Print and shaded views of the part. All mm, measured from the part's lowest x, y and z. Round coordinates to 2 decimals unless told otherwise and drop trailing zeros. Write each loop counter-clockwise with the first axis right and the second up, starting at its lowest first coordinate (ties: lowest second). Pieces come first, ordered by that corner, then holes. Notation, with made-up numbers: (29.25, -7.5) - (86.25, -7.5) arc R10 cw to (86.25, 9.5) - close; hole circle Ø2 at (66.25, 32.25). An arc over 180 degrees is marked (long way). One line per item, written item: value.
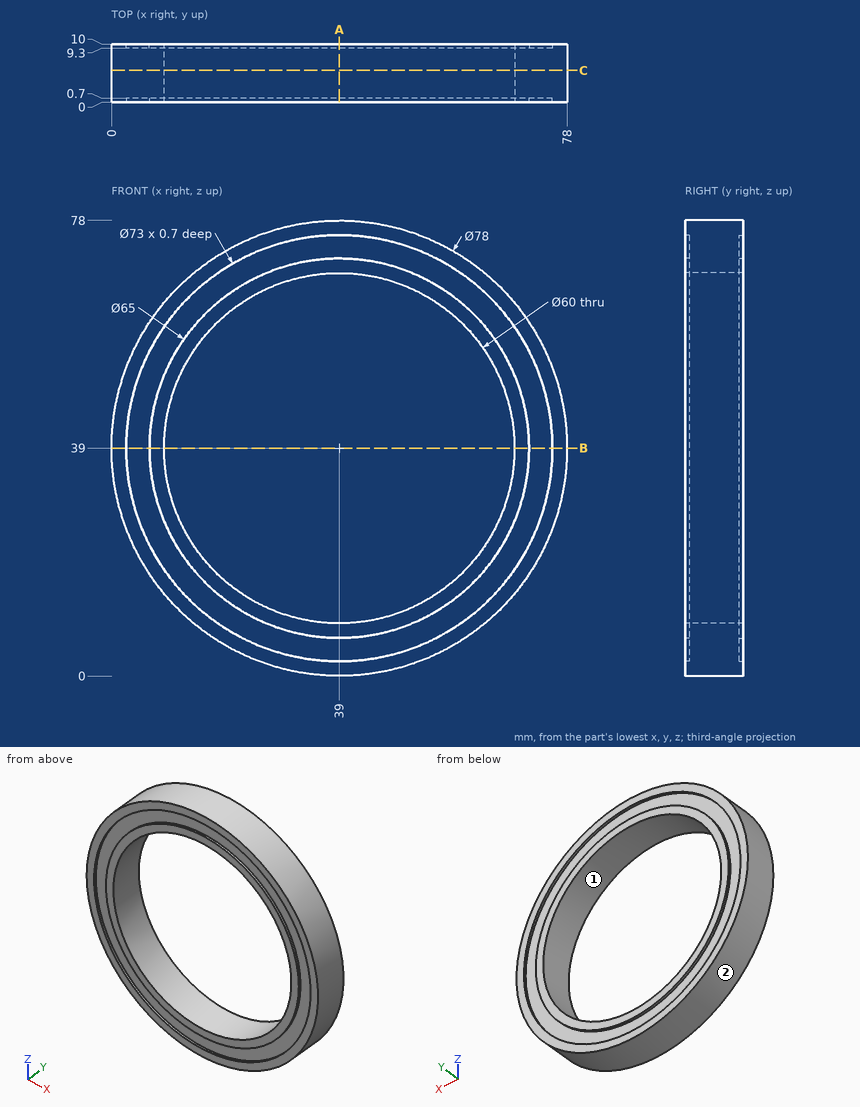
1. Band-saw the part on A-A on x = 39. Write the cut outline in (y, z), plus the area to 3 significant figures.
Report:
outline: (0, 0) - (10, 0) - (10, 2.5) - (9.3, 2.5) - (9.3, 6.5) - (10, 6.5) - (10, 9) - (0, 9) - (0, 6.5) - (0.7, 6.5) - (0.7, 2.5) - (0, 2.5) - close; (0, 69) - (10, 69) - (10, 71.5) - (9.3, 71.5) - (9.3, 75.5) - (10, 75.5) - (10, 78) - (0, 78) - (0, 75.5) - (0.7, 75.5) - (0.7, 71.5) - (0, 71.5) - close
area: 169 mm²
2. Band-saw the part on B-B on z = 39. Write the cut outline in (x, y).
Report:
outline: (0, 0) - (2.5, 0) - (2.5, 0.7) - (6.5, 0.7) - (6.5, 0) - (9, 0) - (9, 10) - (6.5, 10) - (6.5, 9.3) - (2.5, 9.3) - (2.5, 10) - (0, 10) - close; (69, 0) - (71.5, 0) - (71.5, 0.7) - (75.5, 0.7) - (75.5, 0) - (78, 0) - (78, 10) - (75.5, 10) - (75.5, 9.3) - (71.5, 9.3) - (71.5, 10) - (69, 10) - close
3. Mould opens along X. For the marked faces 1 and 2 say: released by +X, released by -X, zero draft, split by the parting line, or undercut.
Report:
face 1: undercut
face 2: split by the parting line
4. Wall check: probe 1 along Z at (x, y) = (39, 0.45); probe 2 along Y at (x, z) = (72.5, 35); probe 3 along Z at (x, y) = (39, 4.25). Give the ranges that are in metal, low to high. Write a range as [from, to].
Report:
probe 1: [0, 2.5], [6.5, 9], [69, 71.5], [75.5, 78]
probe 2: [0.7, 9.3]
probe 3: [0, 9], [69, 78]
5. Band-saw the part on C-C on y = 5.5. Write the cut outline in (x, z), plus the area to 3 significant figures.
Report:
outline: circle Ø78 at (39, 39); hole circle Ø60 at (39, 39)
area: 1,950 mm²
6. Drop flat-ended pins along their axis: pin 1 (4 mm diameter, centred on x = 32, y = 6.5, fed in from +Z); pin 2 (1.5 mm diameter, centred on y = 6, z = 27.5, fed in from +X); pin 3 (2 mm diameter, centred on y = 5, z = 41.5, fed in from -X). Give the stop position or say it passes through.
Report:
pin 1: z = 77.68
pin 2: x = 76.49
pin 3: x = 0.03
